Part print with two shaded views. Sizes in mm from the minimum x, y, z corner. A direction names the side the tool comes from. Coordinates: 2 decimals unless noted, no trailing zeros. Order: outer loops, then holes, each group sorted by start corner. A loop starts at its lowest first (then second) coordinate and runs counter-clockwise, first axis right, second up. Notation, with made-up numbers: (1, -40) - (11, -40) arc R34 ccw to (11, -1) - close; hole circle Ø11 at (29, 87). An arc over 180 degrees is marked (long way). Write each question's results on one line, items separated by ' | '. Start each with the question number.
Q1. Band-saw the part on C-C, the plane x = 475. Write the cut outline in (y, z).
Q2. Wall check: probe 1 along Y at (x, z) = (483, 19.5); probe 2 along Z at (x, y) = (30.5, 29); probe 3 along X at (y, z) = (3, 23). Give the ranges that are in metal, low to high.
Q3. Band-saw the part on A-A, the plane z = 23. Write the cut outline in (x, y), then the cut area to 3 significant figures.
Q4. Which spindle directions (+Z, -Z, +X, -X, +Y, -Y) get a long thin tool onto all of the face, cutting with end or side? Do the marked faces 1, 2 and 3. Say none if no direction does.
Q5. Band-saw the part on B-B, the plane y = 17.5. Write the cut outline in (x, z), then the cut area to 3 significant figures.
Q6. Band-saw the part on D-D, the plane z = 67. Write the cut outline in (x, y), then the cut area to 3 significant figures.
Q7. Pin check, flat tips, straight feed: P1, Ø15, axis at x = 30.5, y = 30, coming from the +Z side; P2, Ø25, axis at x = 20.5, z = 25, coming from the -Y side; P3, Ø25, axis at x = 492, z = 46.5, coming from the +Y side. Stop position of each tip, or through.
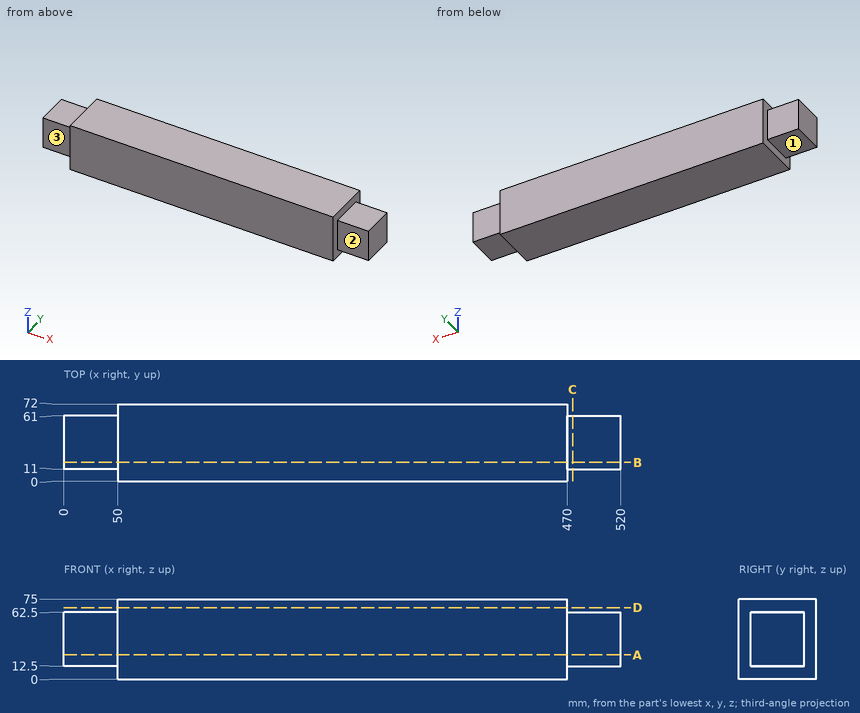
Results below:
1) outline: (11, 12.5) - (61, 12.5) - (61, 62.5) - (11, 62.5) - close
2) probe 1: y = 11 to 61 | probe 2: z = 12.5 to 62.5 | probe 3: x = 50 to 470
3) outline: (0, 11) - (50, 11) - (50, 0) - (470, 0) - (470, 11) - (520, 11) - (520, 61) - (470, 61) - (470, 72) - (50, 72) - (50, 61) - (0, 61) - close | area: 35,200 mm²
4) face 1: -Z, -X, +Y, -Y | face 2: +Z, -Z, +X, -Y | face 3: +Z, -Z, -X, -Y
5) outline: (0, 12.5) - (50, 12.5) - (50, 0) - (470, 0) - (470, 12.5) - (520, 12.5) - (520, 62.5) - (470, 62.5) - (470, 75) - (50, 75) - (50, 62.5) - (0, 62.5) - close | area: 36,500 mm²
6) outline: (50, 0) - (470, 0) - (470, 72) - (50, 72) - close | area: 30,200 mm²
7) P1: stops at z = 62.5 | P2: stops at y = 11 | P3: stops at y = 61
